Verification items for the finished model (mm, model axes). Coordinates: 2 decimals unless noted, no trailing zeros. Write each loop counter-clockwise with the first axis right and the second up, starting at its lowest first coordinate (ties: lowest second). Pieces come first, ordered by that corner, then holes. Notation, with made-up numbers: (35.5, 51.5) -> (78.5, 51.5) arc R15 cw to (78.5, 60.5) -> close; hole circle Ø2 at (55, 26). An arc over 180 degrees is marked (long way). Use a Markdown table: item, result. Add a question column.
Autodesk Inventor part; units mm, degrees
ref_plane "YZ Plane" through (0, 0, 0) normal (1, 0, 0) x (0, 1, 0)
ref_plane "XZ Plane" through (0, 0, 0) normal (0, 1, 0) x (-1, 0, 0)
ref_plane "XY Plane" through (0, 0, 0) normal (0, 0, 1) x (1, 0, 0)
sketch "Sketch1" plane through (0, 0, 0) normal (0, 1, 0) x (-1, 0, 0)
  line L0 (0, 0) -> (660.4, 0)
  line L1 (660.4, 0) -> (660.4, 406.4)
  line L2 (660.4, 406.4) -> (0, 406.4)
  line L3 (0, 406.4) -> (0, 0)
  dimension "d0" = 660.4
  dimension "d1" = 406.4
extrude "Extrusion1" add sketch "Sketch1" along normal blind 3.175
sketch "Sketch2" plane through (0, 3.175, 0) normal (0, 1, 0) x (1, 0, 0)
  line L0 (0, 0) -> (-660.4, 0)
  line L1 (-660.4, 0) -> (-660.4, -406.4)
  line L2 (-660.4, -406.4) -> (0, -406.4)
  line L3 (0, -406.4) -> (0, 0)
  point P0 (-127, -381)
  point P1 (-533.4, -381)
  point P2 (-533.4, -25.4)
  point P3 (-127, -25.4)
  dimension "d4" = 127
  dimension "d5" = 127
  dimension "d6" = 127
  dimension "d7" = 127
  dimension "d8" = 25.4
  dimension "d9" = 25.4
  dimension "d10" = 25.4
  dimension "d11" = 25.4
hole "Hole1" at (-127, 3.175, 381) at (-533.4, 3.175, 381) at (-533.4, 3.175, 25.4) at (-127, 3.175, 25.4) direction (0, -1, 0) diameter 6.35 end through all
sketch "Sketch3" plane through (0, 3.175, 0) normal (0, 1, 0) x (1, 0, 0)
  circle A0 centre (-533.4, -25.4) radius 3.175
  circle A1 centre (-127, -381) radius 3.175
  circle A2 centre (-533.4, -381) radius 3.175
  circle A3 centre (-127, -25.4) radius 3.175
  line L0 (0, 0) -> (-660.4, 0)
  line L1 (-660.4, 0) -> (-660.4, -406.4)
  line L2 (-660.4, -406.4) -> (0, -406.4)
  line L3 (0, -406.4) -> (0, 0)
  point P0 (-127, -228.6)
  point P1 (-127, -177.8)
  point P2 (-533.4, -177.8)
  point P3 (-533.4, -228.6)
  dimension "d19" = 177.8
  dimension "d20" = 177.8
  dimension "d21" = 177.8
  dimension "d22" = 177.8
  dimension "d23" = 127
  dimension "d24" = 127
  dimension "d25" = 127
  dimension "d26" = 127
hole "Hole2" at (-127, 3.175, 228.6) at (-127, 3.175, 177.8) at (-533.4, 3.175, 177.8) at (-533.4, 3.175, 228.6) direction (0, -1, 0) diameter 6.35 end through all
sketch "Sketch4" plane through (0, 3.175, 0) normal (0, 1, 0) x (1, 0, 0)
  circle A0 centre (-533.4, -177.8) radius 3.175
  circle A1 centre (-127, -228.6) radius 3.175
  circle A2 centre (-127, -177.8) radius 3.175
  circle A3 centre (-533.4, -228.6) radius 3.175
  circle A4 centre (-533.4, -25.4) radius 3.175
  circle A5 centre (-127, -381) radius 3.175
  circle A6 centre (-533.4, -381) radius 3.175
  circle A7 centre (-127, -25.4) radius 3.175
  line L0 (0, 0) -> (-660.4, 0)
  line L1 (-660.4, 0) -> (-660.4, -406.4)
  line L2 (-660.4, -406.4) -> (0, -406.4)
  line L3 (0, -406.4) -> (0, 0)
  circle A8 centre (-330.2, -127) radius 9.525
  line L4 (-330.2, -127) -> (-348.1605, -144.9605) construction
  line L5 (-330.2, -127) -> (-304.8, -127) construction
  line L6 (-330.2, -127) -> (-312.2395, -109.0395) construction
  line L7 (-330.2, -127) -> (-304.8, -127) construction
  circle A9 centre (-348.1605, -144.9605) radius 1.9844
  circle A10 centre (-312.2395, -109.0395) radius 1.9844
  dimension "d34" = 19.05
  dimension "d35" = 127
  dimension "d36" = 330.2
  dimension "d37" = 25.4
  dimension "d38" = 135
  dimension "d39" = 25.4
  dimension "d40" = 45
  dimension "d41" = 3.9688
  dimension "d42" = 3.9688
extrude "Extrusion2" cut sketch "Sketch4" against normal blind 3.175 contours A8 | A9 | A10
properties part number "lift plate"
1) Release check for a two-part mould opening along X. For faces 1 (the face through (-337.22, 1.61, 120.56)), 2 (the face through (-326, 3.175, 206)) record: released by +X, released by -X, zero draft, split by the parting line, or undercut.
2) Thickness scan on L1, parallel to X at y = 2.55, z = 381 (3 decimals); L2, parallel to Z at x = -533.4, y = 1.3 (3 decimals); L3, parallel to X at y = 1.55, z = 110. Record the ranges inside material, lowest first.
3) Cross-section at A-A on x = -330.2. Record the boundary of the cut face in (y, z) (3 decimals).
Returned:
| question | item | result |
|---|---|---|
| 1 | face 1 | undercut |
| 1 | face 2 | zero draft |
| 2 | L1 | x = -660.4 to -536.575, -530.225 to -130.175, -123.825 to 0 |
| 2 | L2 | z = 0 to 22.225, 28.575 to 174.625, 180.975 to 225.425, 231.775 to 377.825, 384.175 to 406.4 |
| 2 | L3 | x = -660.4 to -313.98, -310.5 to 0 |
| 3 | outline | (0, 0) -> (3.175, 0) -> (3.175, 117.475) -> (0, 117.475) -> close; (0, 136.525) -> (3.175, 136.525) -> (3.175, 406.4) -> (0, 406.4) -> close |
